```python
from build123d import *

# Parameters (mm, degrees)
SKETCH1_R      = 10.9982
SKETCH1_R_2    = 3.9751
EXTRUDE1_DEPTH = 3.4925
SKETCH2_R      = 9.9822
SKETCH2_R_2    = 4.9911
EXTRUDE2_DEPTH = 0.508


with BuildPart() as part:
    # Sketch1 → Extrude1 (new body)
    with BuildSketch(Plane(origin=(0, 0, 0), x_dir=(0, 0, -1), z_dir=(1, 0, 0))):
        Circle(SKETCH1_R)
        Circle(SKETCH1_R_2, mode=Mode.SUBTRACT)
    extrude1 = extrude(amount=EXTRUDE1_DEPTH)

    # Sketch2 → Extrude2 (cut)
    with BuildSketch(Plane(origin=(3.4925, 0, 0), x_dir=(0, 0, -1), z_dir=(1, 0, 0))):
        Circle(SKETCH2_R)
        Circle(SKETCH2_R_2, mode=Mode.SUBTRACT)
    extrude2 = extrude(amount=-EXTRUDE2_DEPTH, mode=Mode.SUBTRACT)

    # Mirror1: Extrude1, Extrude2 across plane
    add(extrude1.mirror(Plane(origin=(0, 0, 0), x_dir=(0, 0, 1), z_dir=(1, 0, 0))))
    add(extrude2.mirror(Plane(origin=(0, 0, 0), x_dir=(0, 0, 1), z_dir=(1, 0, 0))), mode=Mode.SUBTRACT)


solid = part.part
```
For this review, take the finished solid that the model builds, in its own axes (mm). A direction names the side the tool comes from. Coordinates: 2 decimals unless noted, no trailing zeros. Order: outer loops, then holes, each group sorted by start corner. A loop starts at its lowest first (then second) coordinate and runs counter-clockwise, first axis right, second up. Notation, with made-up numbers: (-23.75, 5) -> (24.25, 5) arc R19 ccw to (24.25, 32) -> close; hole circle Ø10 at (-22.5, 50.5). An arc over 180 degrees is marked (long way). Use CSV: the item, a comma, the result in double quotes. Start each with the question number.
Item 1: Wall thickness on probe 1 along Y at (x, z) = (-2.7, 0); probe 2 along X at (y, z) = (3, 8.25); probe 3 along Z at (x, y) = (-2.25, -1.75): over which ranges is each line inside the solid? List them lowest first.
Item 2: We need section A-A, the plane z = 0. Give the boundary of the cut face in (x, y).
Item 3: We need section D-D, the plane z = -5.25. Give the boundary of the cut face in (x, y).
Item 4: For faces 1 (the face through (3.242, 9.897, 1.299)), 2 (the face through (-3.242, 9.897, 1.299)), 3 (the face through (3.492, -10, -2)), list the 3-axis set-ups (+Z, -Z, +X, -X, +Y, -Y) from which the entire face can be reached by the end or side of a thin tool; tool diameter is ignored.
Item 5: We need section C-C, the plane y = -6.75. Give the boundary of the cut face in (x, z), then the cut area to 3 significant figures.
Item 6: Insertion check: pin 1 (1.5 mm diameter, centred on x = -0.5, y = -1, fed in from +Z); pin 2 (3 mm diameter, centred on x = 0.5, y = 5, fed in from +Z); pin 3 (1.5 mm diameter, centred on x = 0.5, y = -6.5, fed in from -Z). Each pin has a flat end and moves straight along its axis. Give the tip position at first contact, or say it passes through.
Item 7: Draft analysis for pull direction Y (two halves, no side actions). For faces 4 (the face through (0.05, -6.69, 8.73)), 5 (the face through (3.492, -4, 2)), 6 (the face through (3.24, 4.95, 0.65)), state which applies: pulls with the +Y half, pulls with the -Y half, needs draft (parallel to the pull), parting line crosses it, or undercut.
Derived:
1,probe 1,"y = -11 to -3.98, 3.98 to 11"
1,probe 2,"x = -2.98 to 2.98"
1,probe 3,"z = -10.86 to -3.57, 3.57 to 10.86"
2,outline,"(-3.49, -11) -> (3.49, -11) -> (3.49, -9.98) -> (2.98, -9.98) -> (2.98, -4.99) -> (3.49, -4.99) -> (3.49, -3.98) -> (-3.49, -3.98) -> (-3.49, -4.99) -> (-2.98, -4.99) -> (-2.98, -9.98) -> (-3.49, -9.98) -> close; (-3.49, 3.98) -> (3.49, 3.98) -> (3.49, 4.99) -> (2.98, 4.99) -> (2.98, 9.98) -> (3.49, 9.98) -> (3.49, 11) -> (-3.49, 11) -> (-3.49, 9.98) -> (-2.98, 9.98) -> (-2.98, 4.99) -> (-3.49, 4.99) -> close"
3,outline,"(-3.49, -9.66) -> (3.49, -9.66) -> (3.49, -8.49) -> (2.98, -8.49) -> (2.98, 8.49) -> (3.49, 8.49) -> (3.49, 9.66) -> (-3.49, 9.66) -> (-3.49, 8.49) -> (-2.98, 8.49) -> (-2.98, -8.49) -> (-3.49, -8.49) -> close"
4,face 1,"+X"
4,face 2,"-X"
4,face 3,"+Z, -Z, +X, +Y, -Y"
5,outline,"(-3.49, -8.68) -> (3.49, -8.68) -> (3.49, -7.35) -> (2.98, -7.35) -> (2.98, 7.35) -> (3.49, 7.35) -> (3.49, 8.68) -> (-3.49, 8.68) -> (-3.49, 7.35) -> (-2.98, 7.35) -> (-2.98, -7.35) -> (-3.49, -7.35) -> close"
5,area,"106 mm^2"
6,pin 1,"stops at z = 11"
6,pin 2,"stops at z = 10.43"
6,pin 3,"stops at z = -9.38"
7,face 4,"parting line crosses it"
7,face 5,"needs draft"
7,face 6,"undercut"
